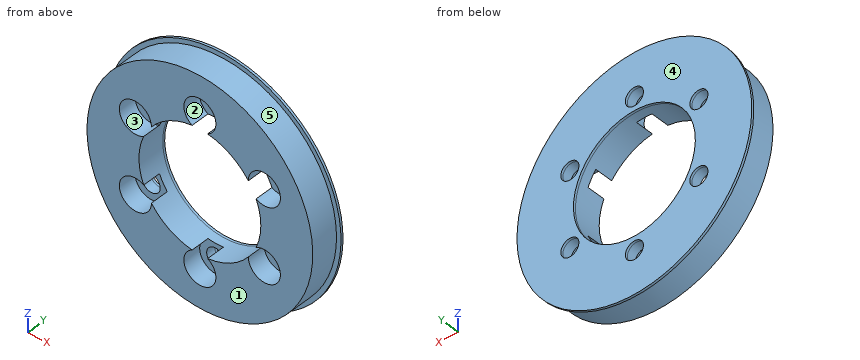
from build123d import *

# Parameters (mm, degrees)
SKETCH1_R           = 25
SKETCH1_R_2         = 13.5
BOSS_EXTRUDE1_DEPTH = 6
SKETCH2_R           = 2
CUT_EXTRUDE1_DEPTH  = 36.860842154
SKETCH3_R           = 3.55
CUT_EXTRUDE4_DEPTH  = 4
CIRPATTERN2_COUNT   = 6
SKETCH4_R           = 26
SKETCH4_R_2         = 2
SKETCH4_R_3         = 13.5
BOSS_EXTRUDE3_DEPTH = 0.5


with BuildPart() as part:
    # Sketch1 → Boss-Extrude1 (new body)
    with BuildSketch(Plane(origin=(0, 0, 0), x_dir=(1, 0, 0), z_dir=(0, 1, 0))):
        with Locations(Location((0, 0, 0), (0, 0, 270))):
            Circle(SKETCH1_R)
        with Locations(Location((0, 0, 0), (0, 0, 270))):
            Circle(SKETCH1_R_2, mode=Mode.SUBTRACT)
    extrude(amount=BOSS_EXTRUDE1_DEPTH)

    # Sketch2 → Cut-Extrude1 (cut, through all)
    with BuildSketch(Plane(origin=(0, 6, 0), x_dir=(1, 0, 0), z_dir=(0, 1, 0))):
        with Locations(Location((0, 16.5, 0), (0, 0, 270))):
            Circle(SKETCH2_R)
    cut_extrude1 = extrude(amount=-CUT_EXTRUDE1_DEPTH, mode=Mode.SUBTRACT)

    # Sketch3 → Cut-Extrude4 (cut)
    with BuildSketch(Plane(origin=(0, 0, 0), x_dir=(1, 0, 0), z_dir=(0, 1, 0))):
        with Locations((0, 16.5)):
            Circle(SKETCH3_R)
    cut_extrude4 = extrude(amount=CUT_EXTRUDE4_DEPTH, mode=Mode.SUBTRACT)

    # CirPattern2: Cut-Extrude1, Cut-Extrude4 ×6 about axis
    cirpattern2_axis = Axis((0, 0, 0), (0, 1, 0))
    add([cut_extrude1.rotate(cirpattern2_axis, i * 360 / CIRPATTERN2_COUNT) for i in range(1, CIRPATTERN2_COUNT)], mode=Mode.SUBTRACT)
    add([cut_extrude4.rotate(cirpattern2_axis, i * 360 / CIRPATTERN2_COUNT) for i in range(1, CIRPATTERN2_COUNT)], mode=Mode.SUBTRACT)

    # Sketch4 → Boss-Extrude3 (add)
    with BuildSketch(Plane(origin=(0, 6, 0), x_dir=(1, 0, 0), z_dir=(0, 1, 0))):
        with Locations(Location((0, 0, 0), (0, 0, 270))):
            Circle(SKETCH4_R)
        with Locations(Location((14.289419162, 8.25, 0), (0, 0, 270))):
            Circle(SKETCH4_R_2, mode=Mode.SUBTRACT)
        with Locations(Location((14.289419162, -8.25, 0), (0, 0, 270))):
            Circle(SKETCH4_R_2, mode=Mode.SUBTRACT)
        with Locations(Location((0, -16.5, 0), (0, 0, 270))):
            Circle(SKETCH4_R_2, mode=Mode.SUBTRACT)
        with Locations(Location((0, 0, 0), (0, 0, 82.708634602))):
            Circle(SKETCH4_R_3, mode=Mode.SUBTRACT)
        with Locations(Location((-14.289419162, -8.25, 0), (0, 0, 270))):
            Circle(SKETCH4_R_2, mode=Mode.SUBTRACT)
        with Locations(Location((-14.289419162, 8.25, 0), (0, 0, 270))):
            Circle(SKETCH4_R_2, mode=Mode.SUBTRACT)
        with Locations(Location((0, 16.5, 0), (0, 0, 270))):
            Circle(SKETCH4_R_2, mode=Mode.SUBTRACT)
    extrude(amount=BOSS_EXTRUDE3_DEPTH)


solid = part.part
Model file for the job. Use its own axes, mm. Face numbers are marked on the shaded views. A direction names the side the tool comes from. Give positions to 0.01 mm unless a question says otherwise; leave off trailing zeros. Loops run counter-clockwise (first coordinate to the right, second up) from the corner with the lowest first, then second, coordinate; pieces in that order, holes last. Notation, with made-up numbers: (72, 5.25) -> (92, 5.25) arc R19 cw to (92, 38.25) -> close; hole circle Ø6 at (4.5, -39.75). An arc over 180 degrees is marked (long way). Use a Markdown table: item, result. Add a question column.
(1) Tool access for the marked faces 1 and 2: list every direction of +Z, -Z, +X, -X, +Y, -Y with a clear straight run to the whole face (end or side of a thin tool).
(2) Slice it at C-C on x = 10. List the corners of the cut face in (y, z).
(3) Drop flat-ended pins along their axis: pin 1 Ø5.5 at (x, z) = (-13.5, -7) entering from -Y; pin 2 Ø1 at (y, z) = (3.5, 11.5) entering from -X; pin 3 Ø2 at (x, z) = (-13, 9) entering from -Y; pin 4 Ø3.5 at (x, z) = (-14.29, 8.25) entering from +Y. Give the stop position or say it passes through.
(4) Slice it at A-A on x = 0. List the corners of the cut face in (y, z), and give its area (3 significant figures).
(5) Slice it at D-D on y = 2. List the corners of the cut face in (x, z).
(6) Mould opens along Z. For the marked faces 3, 4 and 5 say: +Z half, -Z half, draft (parallel to the pull), parting line (faces both ways), or undercut.
(7) Wall check: line 1 along X through (y, z) = (2.2, 0); line 2 along X through (y, z) = (5.55, 8.25); line 3 along X through (y, z) = (6.35, -8.25). Give the ranges that are in metal, low to high.
(8) Slice it at B-B on z = 11. List the corners of the cut face in (x, y).
Filled sheet:
| question | item | result |
|---|---|---|
| 1 | face 1 | +Z, -Z, +X, -X, -Y |
| 1 | face 2 | -Y |
| 2 | outline | (0, -22.91) -> (6, -22.91) -> (6, -24) -> (6.5, -24) -> (6.5, -9.07) -> (0, -9.07) -> close; (0, 9.07) -> (6.5, 9.07) -> (6.5, 24) -> (6, 24) -> (6, 22.91) -> (0, 22.91) -> close |
| 3 | pin 1 | y = 0 |
| 3 | pin 2 | x = -22.45 |
| 3 | pin 3 | y = 4 |
| 3 | pin 4 | through |
| 4 | outline | (0, -25) -> (6, -25) -> (6, -26) -> (6.5, -26) -> (6.5, -18.5) -> (4, -18.5) -> (4, -20.05) -> (0, -20.05) -> close; (0, 20.05) -> (4, 20.05) -> (4, 18.5) -> (6.5, 18.5) -> (6.5, 26) -> (6, 26) -> (6, 25) -> (0, 25) -> close; (4, -14.5) -> (6.5, -14.5) -> (6.5, -13.5) -> (4, -13.5) -> close; (4, 13.5) -> (6.5, 13.5) -> (6.5, 14.5) -> (4, 14.5) -> close |
| 4 | area | 78.1 mm2 |
| 5 | outline | circle Ø50 at (0, 0); hole (-12.45, -5.21) arc R3.55 ccw (long way) to (-10.74, -8.18) arc R13.5 ccw to (-1.71, -13.39) arc R3.55 ccw (long way) to (1.71, -13.39) arc R13.5 ccw to (10.74, -8.18) arc R3.55 ccw (long way) to (12.45, -5.21) arc R13.5 ccw to (12.45, 5.21) arc R3.55 ccw (long way) to (10.74, 8.18) arc R13.5 ccw to (1.71, 13.39) arc R3.55 ccw (long way) to (-1.71, 13.39) arc R13.5 ccw to (-10.74, 8.18) arc R3.55 ccw (long way) to (-12.45, 5.21) arc R13.5 ccw to start |
| 6 | face 3 | undercut |
| 6 | face 4 | draft |
| 6 | face 5 | parting line |
| 7 | line 1 | -25 to -13.5, 13.5 to 25 |
| 7 | line 2 | -23.6 to -16.29, -12.29 to -10.69, 10.69 to 12.29, 16.29 to 23.6 |
| 7 | line 3 | -24.66 to -16.29, -12.29 to -10.69, 10.69 to 12.29, 16.29 to 24.66 |
| 8 | outline | (-23.56, 6) -> (-22.45, 6) -> (-22.45, 0) -> (-16.53, 0) -> (-16.53, 4) -> (-12.04, 4) -> (-12.04, 0) -> (-7.83, 0) -> (-7.83, 6.5) -> (-23.56, 6.5) -> close; (7.83, 0) -> (12.04, 0) -> (12.04, 4) -> (16.53, 4) -> (16.53, 0) -> (22.45, 0) -> (22.45, 6) -> (23.56, 6) -> (23.56, 6.5) -> (7.83, 6.5) -> close |
